Geometry check sheet. Reference: the model listing, model coordinates, mm. Face numbers are marked on the shaded views. A direction names the side the tool comes from. Coordinates: 2 decimals unless noted, no trailing zeros. Order: outer loops, then holes, each group sorted by start corner. A loop starts at its lowest first (then second) coordinate and runs counter-clockwise, first axis right, second up. Notation, with made-up numbers: M 89,-15 L 103,-15 A21 ccw 103,14 Z; hole C 39,9 d9. An arc over 180 degrees is marked long. One line per item, written item: value. Start each with the question number.
1) Sectioned sample at C-C, the plane z = -3. Enter the section's corners in (x, y), then the cut area to 3 significant figures.
2) Sectioned sample at A-A, the plane x = 0. Enter the section's corners in (y, z).
3) Go/stop test with flat-tipped pins: P1, Ø12, axis at x = -8.5, z = 12, coming from the +Y side; P2, Ø9, axis at x = -34, z = 5.5, coming from the -Y side; P3, Ø1.5, axis at y = -15, z = 4, coming from the +X side. Record where each tip stops, or that it passes through.
4) Thickness scan on L1, parallel to X at y = -1, z = 3.25; L2, parallel to Y at x = -2.5, z = -2.75; L3, parallel to X at y = -9, z = 16.25. Record the ranges inside material, lowest first. Write a range as from..to.
5) Access from +Z, -Z, +X, -X, +Y, -Y to the whole of each face (thin tool, end or side, straight path). Record for the marked faces 1 and 2.
6) Sectioned sample at B-B, the plane z = 10.75. Enter the section's corners in (x, y).
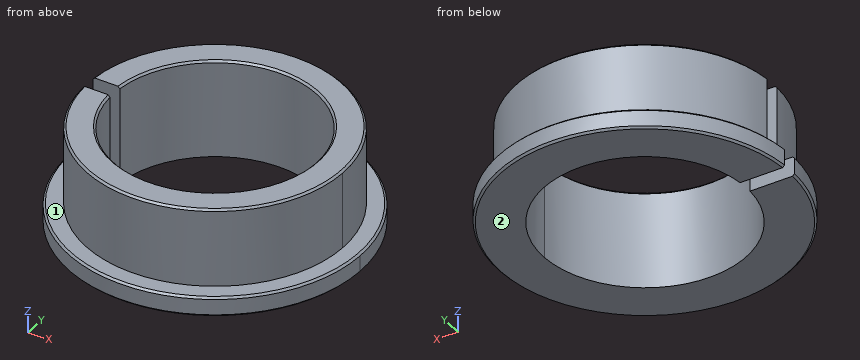
```python
from build123d import *

# Parameters (mm, degrees)
F0_R     = 33
F0_R_2   = 26
F1_DEPTH = 20
F2_R     = 37.5
F2_R_2   = 26
F3_DEPTH = 5
F4_W     = 22
F4_H     = 4
F5_DEPTH = 25
F6_SIZE  = 0.5


with BuildPart() as f1:
    # F0 (on Top) → F1 (new body)
    with BuildSketch(Plane.XY):
        Circle(F0_R)
        Circle(F0_R_2, mode=Mode.SUBTRACT)
    extrude(amount=F1_DEPTH)

    # F2 (on Top) → F3 (join)
    with BuildSketch(Plane.XY):
        Circle(F2_R)
        Circle(F2_R_2, mode=Mode.SUBTRACT)
    extrude(amount=-F3_DEPTH)

    # F4 (on Top) → F5 (cut, symmetric)
    with BuildSketch(Plane.XY):
        with Locations((-31.949636, 0)):
            Rectangle(F4_W, F4_H)
    extrude(amount=F5_DEPTH, both=True, mode=Mode.SUBTRACT)

    # F6
    f6_edges = [f1.edges().sort_by_distance(p)[0] for p in [
        (1.00046, 32.984831, 20),
        (1.00046, -32.984831, 20),
        (1.000742, -25.980734, 20),
        (1.000742, 25.980734, 20),
        (1.000356, -37.486655, 0),
        (1.000356, 37.486655, 0),
        (1.000356, -37.486655, -5),
        (1.000356, 37.486655, -5),
    ]]
    chamfer(f6_edges, length=F6_SIZE)


solid = f1.part
```
Final values:
1. outline: M -37.45,-2 A37.5 ccw long -37.45,2 L -25.92,2 A26 cw long -25.92,-2 Z
1. area: 2,250 mm^2
2. outline: M -37.5,-4.5 L -37,-5 L -26,-5 L -26,19.5 L -26.5,20 L -32.5,20 L -33,19.5 L -33,0 L -37,0 L -37.5,-0.5 Z; M 26,-5 L 37,-5 L 37.5,-4.5 L 37.5,-0.5 L 37,0 L 33,0 L 33,19.5 L 32.5,20 L 26.5,20 L 26,19.5 Z
3. P1: stops at y = 32.91
3. P2: stops at y = -14.79
3. P3: stops at x = 29.76
4. L1: x = 25.98..32.98
4. L2: y = -37.42..-25.88, 25.88..37.42
4. L3: x = -31.75..-24.39, 24.39..31.75
5. face 1: +Z
5. face 2: -Z, +X, -X, +Y, -Y
6. outline: M -32.94,-2 A33 ccw long -32.94,2 L -25.92,2 A26 cw long -25.92,-2 Z
